Autodesk Inventor part; units mm, degrees
ref_plane "YZ Plane" through (0, 0, 0) normal (1, 0, 0) x (0, 1, 0)
ref_plane "XZ Plane" through (0, 0, 0) normal (0, 1, 0) x (-1, 0, 0)
ref_plane "XY Plane" through (0, 0, 0) normal (0, 0, 1) x (1, 0, 0)
sketch "Sketch1" plane through (0, 0, 0) normal (1, 0, 0) x (0, 1, 0)
  line L0 (0, 0) -> (-114.3, 0)
  line L1 (-114.3, 0) -> (-114.3, -444.5)
  line L2 (-114.3, -444.5) -> (0, -444.5)
  line L3 (-114.3, 0) -> (-25.4, 0)
  line L4 (-25.4, 0) -> (-25.4, -117.6782)
  line L5 (-25.4, -117.6782) -> (-114.3, -117.6782)
  line L6 (-114.3, -117.6782) -> (-114.3, 0)
  line L7 (-114.3, -444.5) -> (-25.4, -444.5)
  line L8 (-25.4, -444.5) -> (-25.4, -326.8218)
  line L9 (-25.4, -326.8218) -> (-114.3, -326.8218)
  line L10 (-114.3, -326.8218) -> (-114.3, -444.5)
  line L11 (-25.4, -143.0782) -> (-88.9, -143.0782)
  line L12 (-88.9, -143.0782) -> (-88.9, -301.4218)
  line L13 (-88.9, -301.4218) -> (-25.4, -301.4218)
  line L14 (-25.4, -301.4218) -> (-25.4, -143.0782)
  line L15 (279.4, -117.6782) -> (279.4, -326.8218)
  line L16 (-114.3, -326.8218) -> (-114.3, -117.6782)
  line L17 (0, -143.0782) -> (254, -143.0782)
  line L18 (254, -143.0782) -> (254, -301.4218)
  line L19 (254, -301.4218) -> (0, -301.4218)
  line L20 (0, -301.4218) -> (0, -143.0782)
  line L21 (0, -117.6782) -> (0, 0)
  line L22 (0, -444.5) -> (0, -326.8218)
  line L23 (0, -301.4218) -> (0, -143.0782)
  line L24 (-114.3, -117.6782) -> (-25.4, -117.6782)
  line L25 (0, -117.6782) -> (254, -117.6782)
  line L26 (254, -326.8218) -> (0, -326.8218)
  line L27 (-25.4, -326.8218) -> (-114.3, -326.8218)
  line L28 (254, -326.8218) -> (254, -444.5)
  line L29 (254, -444.5) -> (279.4, -444.5)
  line L30 (279.4, -444.5) -> (279.4, -326.8218)
  line L31 (254, -117.6782) -> (254, 0)
  line L32 (254, 0) -> (279.4, 0)
  line L33 (279.4, 0) -> (279.4, -117.6782)
  dimension "d0" = 114.3
  dimension "d1" = 444.5
  dimension "d2" = 88.9
  dimension "d3" = 209.1436
  dimension "d4" = 117.6782
  dimension "d9" = 63.5
  dimension "d10" = 158.3436
  dimension "d11" = 25.4
  dimension "d12" = 25.4
  dimension "d16" = 254
  dimension "d24" = 117.6782
  dimension "d25" = 25.4
  dimension "d26" = 117.6782
  dimension "d27" = 25.4
  dimension "d28" = 393.7
extrude "Extrusion2" add sketch "Sketch1" along normal blind 6.35 contours L21 L25 L31 L32 L33 L15 L30 L29 L28 L26 L22 L2 L8 L9 L1 L5 L4 L0
properties part number "CapBallLiftBacking"
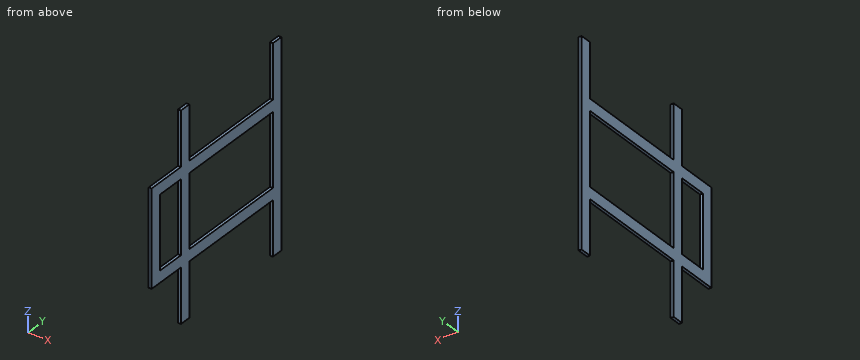
Could you check a few things on this model? Use its own coordinates, in mm. Round coordinates to 2 decimals unless told otherwise and drop trailing zeros. Write each loop counter-clockwise with the first axis right and the second up, starting at its lowest first coordinate (ties: lowest second). Pieces come first, ordered by that corner, then holes. Notation, with made-up numbers: (33, 63.5) - (54, 63.5) arc R24 cw to (54, 76.5) - close; hole circle Ø1 at (42, 34). An arc over 180 degrees is marked (long way). Put each result on its own line as item: value. Start each with the question number.
(1) Will these pins go through, and if not, where does the flat tip stop? pin 1 (3 mm diameter, centred on x = 4.5, y = -52, fed in from -Z); pin 2 (3 mm diameter, centred on x = 4, y = -50, fed in from +Z); pin 3 (1.9 mm diameter, centred on x = 2, z = -385.5, fed in from -Y).
(2) I want a section at A-A, the plane y = 44. Please give me the cut outline in (x, z), plus the area to 3 significant figures.
(3) I want a section at B-B, the plane x = 3.75. Please give me the cut outline in (y, z), plus the area to 3 significant figures.
(4) I want a section at D-D, the plane z = -238.5. Please give me the cut outline in (x, y), plus the area to 3 significant figures.
(5) I need wall thicknesses on probe 1 along Y at (x, z) = (0.5, -298); probe 2 along Y at (x, z) = (4.75, -346.5); probe 3 along Z at (x, y) = (0.75, 240.5). Which ranges of each line are inside material? Lowest first, please.
(6) I want a section at C-C, the plane z = -64. Please give me the cut outline in (x, y).
Here are the results:
1. pin 1: stops at z = -326.82
1. pin 2: stops at z = -117.68
1. pin 3: stops at y = -25.4
2. outline: (0, -326.82) - (6.35, -326.82) - (6.35, -301.42) - (0, -301.42) - close; (0, -143.08) - (6.35, -143.08) - (6.35, -117.68) - (0, -117.68) - close
2. area: 323 mm^2
3. outline: (-114.3, -326.82) - (-25.4, -326.82) - (-25.4, -444.5) - (0, -444.5) - (0, -326.82) - (254, -326.82) - (254, -444.5) - (279.4, -444.5) - (279.4, 0) - (254, 0) - (254, -117.68) - (0, -117.68) - (0, 0) - (-25.4, 0) - (-25.4, -117.68) - (-114.3, -117.68) - close; hole (-88.9, -301.42) - (-25.4, -301.42) - (-25.4, -143.08) - (-88.9, -143.08) - close; hole (0, -301.42) - (254, -301.42) - (254, -143.08) - (0, -143.08) - close
3. area: 44,000 mm^2
4. outline: (0, -114.3) - (6.35, -114.3) - (6.35, -88.9) - (0, -88.9) - close; (0, -25.4) - (6.35, -25.4) - (6.35, 0) - (0, 0) - close; (0, 254) - (6.35, 254) - (6.35, 279.4) - (0, 279.4) - close
4. area: 484 mm^2
5. probe 1: y = -114.3 to -88.9, -25.4 to 0, 254 to 279.4
5. probe 2: y = -25.4 to 0, 254 to 279.4
5. probe 3: z = -326.82 to -301.42, -143.08 to -117.68
6. outline: (0, -25.4) - (6.35, -25.4) - (6.35, 0) - (0, 0) - close; (0, 254) - (6.35, 254) - (6.35, 279.4) - (0, 279.4) - close
